from build123d import *

# Parameters (mm, degrees)
BOSS_EXTRUDE1_DEPTH  = 4.125
BOSS_EXTRUDE2_START  = 2
BOSS_EXTRUDE2_DEPTH  = 2
SKETCH3_R            = 1.7
SKETCH3_R_2          = 1.5
BOSS_EXTRUDE3_DEPTH  = 4
BOSS_EXTRUDE4_DEPTH  = 4.125
FILLET2_R            = 2.5
SKETCH9_R            = 3.5
CUT_EXTRUDE1_DEPTH   = 99.03896228
SKETCH10_R           = 12.5
SKETCH10_R_2         = 7.5
BOSS_EXTRUDE9_DEPTH  = 4.125
BOSS_EXTRUDE11_DEPTH = 2
BOSS_EXTRUDE12_DEPTH = 4


with BuildPart() as part:
    # Sketch1 → Boss-Extrude1 (new body)
    with BuildSketch(Plane.XY):
        with BuildLine():
            Line((0, 0), (14, 0))
            ThreePointArc((14, 0), (17.925, 3.925), (14, 7.85))
            Line((14, 7.85), (0, 7.85))
            Line((0, 7.85), (0, 12.85))
            Line((0, 12.85), (14, 12.85))
            ThreePointArc((14, 12.85), (22.925, 3.925), (14, -5))
            Line((14, -5), (0, -5))
            Line((0, -5), (0, 0))
        make_face()
    extrude(amount=BOSS_EXTRUDE1_DEPTH)

    # Sketch2 → Boss-Extrude2 (add)
    with BuildSketch(Plane(origin=(0, 0, 0), x_dir=(-1, 0, 0), z_dir=(0, 0, -1)).offset(BOSS_EXTRUDE2_START)):
        with BuildLine():
            Line((-14, 6.7375), (0, 6.7375))
            Line((0, 6.7375), (0, 7.85))
            Line((0, 7.85), (0, 12.85))
            Line((0, 12.85), (-14, 12.85))
            ThreePointArc((-14, 12.85), (-22.925, 3.925), (-14, -5))
            Line((-14, -5), (0, -5))
            Line((0, -5), (0, 0))
            Line((0, 0), (0, 1.1125))
            Line((0, 1.1125), (-14, 1.1125))
            ThreePointArc((-14, 1.1125), (-16.8125, 3.925), (-14, 6.7375))
        make_face()
    extrude(amount=-BOSS_EXTRUDE2_DEPTH)

    # Sketch3 → Boss-Extrude3 (add)
    with BuildSketch(Plane.XY.offset(4.125)):
        with BuildLine():
            Line((0, 12.85), (-3.238869072, 12.85))
            ThreePointArc((-3.238869072, 12.85), (-5.006636025, 12.117766953), (-5.738869072, 10.35))
            Line((-5.738869072, 10.35), (-5.738869072, -2.5))
            ThreePointArc((-5.738869072, -2.5), (-5.006636025, -4.267766953), (-3.238869072, -5))
            Line((-3.238869072, -5), (0, -5))
            Line((0, -5), (14, -5))
            ThreePointArc((14, -5), (18.764286268, -3.621999494), (22.057381748, 0.086481488))
            Line((22.057381748, 0.086481488), (22.057381748, 7.763518512))
            ThreePointArc((22.057381748, 7.763518512), (18.764286268, 11.471999494), (14, 12.85))
            Line((14, 12.85), (0, 12.85))
        make_face()
        with Locations((14, 3.8625)):
            Circle(SKETCH3_R, mode=Mode.SUBTRACT)
        with Locations((10, 3.8625)):
            Circle(SKETCH3_R, mode=Mode.SUBTRACT)
        with Locations((-1, 3.8625)):
            Circle(SKETCH3_R_2, mode=Mode.SUBTRACT)
    extrude(amount=BOSS_EXTRUDE3_DEPTH)

    # Sketch4 → Boss-Extrude4 (add)
    with BuildSketch(Plane.XY):
        with BuildLine():
            Line((89.5, 11.3625), (18.721642326, 11.3625))
            ThreePointArc((18.721642326, 11.3625), (22.8625, 3.8625), (18.721642326, -3.6375))
            Line((18.721642326, -3.6375), (89.5, -3.6375))
            ThreePointArc((89.5, -3.6375), (97, 3.8625), (89.5, 11.3625))
        make_face()
    extrude(amount=BOSS_EXTRUDE4_DEPTH)

    # Fillet2
    # the kernel refuses this fillet: 2.5 mm, written as the material it adds along each edge
    with BuildSketch(Plane(origin=(18.739643315, -3.6375, 4.125), x_dir=(1, 0, 0), z_dir=(0, 0, -1))) as fillet2_piece_1:
        with BuildLine():
            CenterArc((0.671153184, 2.5), FILLET2_R, 241.732240209, 28.267759791)
            ThreePointArc((-0.512828544, 0.298140044), (-0.253936624, 0.153331807), (0, 0))
            Line((0, 0), (0.671153184, 0))
        make_face()
    extrude(amount=4.125)
    with BuildSketch(Plane(origin=(18.933479376, 11.3625, 4.125), x_dir=(1, 0, 0), z_dir=(0, 0, -1))) as fillet2_piece_2:
        with BuildLine():
            CenterArc((0.703604866, -2.5), FILLET2_R, 90, 29.564237734)
            ThreePointArc((-0.52989278, -0.325492341), (-0.262110566, -0.167362816), (0, 0))
            Line((0, 0), (0.703604866, 0))
        make_face()
    extrude(amount=4.125)

    # Sketch9 → Cut-Extrude1 (cut, through all)
    with BuildSketch(Plane.XY.offset(4.125)):
        with Locations((89.5, 3.8625)):
            Circle(SKETCH9_R)
    extrude(amount=-CUT_EXTRUDE1_DEPTH, mode=Mode.SUBTRACT)

    # Sketch10 → Boss-Extrude9 (add)
    with BuildSketch(Plane(origin=(0, 0, 0), x_dir=(-1, 0, 0), z_dir=(0, 0, -1))):
        with Locations((-89.5, 3.8625)):
            Circle(SKETCH10_R)
        with Locations((-89.5, 3.8625)):
            Circle(SKETCH10_R_2, mode=Mode.SUBTRACT)
    extrude(amount=-BOSS_EXTRUDE9_DEPTH)

    # Sketch12 → Boss-Extrude11 (add)
    with BuildSketch(Plane(origin=(0, 0, 0), x_dir=(-1, 0, 0), z_dir=(0, 0, -1))):
        with BuildLine():
            Line((-19.637084242, 11.3625), (-67.931783013, 11.3625))
            ThreePointArc((-67.931783013, 11.3625), (-69.959582845, 3.85224622), (-67.857301806, -3.6375))
            Line((-67.857301806, -3.6375), (-19.410796499, -3.6375))
            ThreePointArc((-19.410796499, -3.6375), (-18.800325324, -3.713180519), (-18.22681477, -3.935640044))
            ThreePointArc((-18.22681477, -3.935640044), (-22.924428786, 3.824025558), (-18.403586596, 11.687992341))
            ThreePointArc((-18.403586596, 11.687992341), (-18.999224205, 11.445242344), (-19.637084242, 11.3625))
        make_face()
    extrude(amount=BOSS_EXTRUDE11_DEPTH)

    # Sketch13 → Boss-Extrude12 (add)
    with BuildSketch(Plane.XY.offset(4.125)):
        with BuildLine():
            Line((67.931783013, 11.3625), (19.637084242, 11.3625))
            ThreePointArc((19.637084242, 11.3625), (18.999224205, 11.445242344), (18.403586596, 11.687992341))
            ThreePointArc((18.403586596, 11.687992341), (20.532174732, 10.006637795), (22.057381748, 7.763518512))
            Line((22.057381748, 7.763518512), (22.057381748, 0.086481488))
            ThreePointArc((22.057381748, 0.086481488), (20.462951062, -2.230151385), (18.22681477, -3.935640044))
            ThreePointArc((18.22681477, -3.935640044), (18.800325324, -3.713180519), (19.410796499, -3.6375))
            Line((19.410796499, -3.6375), (67.857301806, -3.6375))
            ThreePointArc((67.857301806, -3.6375), (69.959582845, 3.85224622), (67.931783013, 11.3625))
        make_face()
    extrude(amount=BOSS_EXTRUDE12_DEPTH)


solid = part.part
Verification items for the finished model (mm, model axes). A direction names the side the tool comes from. Give positions to 0.01 mm unless a question says otherwise; leave off trailing zeros. Write each loop counter-clockwise with the first axis right and the second up, starting at its lowest first coordinate (ties: lowest second). Pieces come first, ordered by that corner, then holes. Notation, with made-up numbers: (83, -28) -> (132, -28) arc R13 cw to (132, -23) -> close; hole circle Ø5 at (33, 50). An arc over 180 degrees is marked (long way). Use CSV: the item, a comma, the result in double quotes.
(1) Sectioned sample at C-C (z = 6.5). Give the number of separate pieces and of enclosed holes in the cut face, plus the area to 3 significant figures.
Derived:
separate pieces,"1"
enclosed holes,"3"
area,"1,160 mm^2"
(2) Go/stop test with flat-tipped pins: pin 1 (4.5 mm diameter, centred on x = 14, y = 3.86, fed in from -Z) (3 decimals); pin 2 (3.5 mm diameter, centred on x = 6.5, z = 1.5, fed in from -Y); pin 3 (6 mm diameter, centred on x = 85.5, z = 4, fed in from -Y). Record where each tip stops, or that it passes through.
Derived:
pin 1,"stops at z = 4.125"
pin 2,"stops at y = -5"
pin 3,"stops at y = -8.6"
(3) Sectioned sample at D-D (y = -1). Record the cut outline in (x, z) (3 decimals).
Derived:
outline,"(-5.739, 4.125) -> (0, 4.125) -> (0, -2) -> (69.107, -2) -> (69.107, 0) -> (101.015, 0) -> (101.015, 4.125) -> (69.107, 4.125) -> (69.107, 8.125) -> (-5.739, 8.125) -> close"
(4) Release check for a two-part mould opening along Y. For faces 1 (the cylindrical face through (69.96, 3.74, 6.1)), 2 (the flat face through (7, 0, 2)), 3 (the flat face through (85, 4, 0)) record: +Y half, -Y half, draft (parallel to the pull), parting line (faces both ways), or undercut.
Derived:
face 1,"parting line"
face 2,"undercut"
face 3,"draft"
(5) Material ranges on L1, parallel to Y at x = -1, z = 5.05; L2, parallel to Y at x = 89.5, z = 2.9; L3, parallel to Z at x = 76, y = 7.5 (3 decimals), recorded low to high.
Derived:
L1,"y = -5 to 2.36, 5.36 to 12.85"
L2,"y = -8.64 to 0.36, 7.36 to 16.36"
L3,"z = 0 to 4.125"
(6) Set-up check for faces 4 (the flat face through (7, -5, 3)), 5 (the flat face through (50, 11.362, 3)), 6 (the flat face through (0, 10, 1)), 7 (the flat face through (7, 7.85, 2)): record each of +Z, -Z, +X, -X, +Y, -Y from which the full face is reachable in a straight line by a thin tool's end or side.
Derived:
face 4,"+Z, -Z, -X, -Y"
face 5,"+Z, -Z, +Y"
face 6,"-Z, -X, +Y, -Y"
face 7,"-X"
(7) Sectioned sample at A-A (x = 89.5). Record the cut outline in (y, z) (1 decimal).
Derived:
outline,"(-8.6, 0) -> (0.4, 0) -> (0.4, 4.1) -> (-8.6, 4.1) -> close; (7.4, 0) -> (16.4, 0) -> (16.4, 4.1) -> (7.4, 4.1) -> close"
